Geometry: final body of the model. Coordinates: model frame, mm. A direction names the side the tool comes from. Round coordinates to 2 decimals unless told otherwise and drop trailing zeros. Loops run counter-clockwise (first coordinate to the right, second up) from the corner with the lowest first, then second, coordinate; pieces in that order, holes last. Notation, with made-up numbers: M -21,21 L -12,21 A33 ccw -12,53 Z; hole C 26,2 d8. An arc over 180 degrees is marked long. Answer as a JSON object with one key per item and string values.
from build123d import *

# Parameters (mm, degrees)
SKETCH1_W               = 35
SKETCH1_H               = 12.2
BOSS_EXTRUDE1_DEPTH     = 4
SKETCH2_R               = 1
CUT_EXTRUDE1_DEPTH      = 38.656658625
SKETCH3_W               = 10
SKETCH3_H               = 12.2
BOSS_EXTRUDE2_DEPTH     = 15
SKETCH4_W               = 12.2
SKETCH4_H               = 4
BOSS_EXTRUDE3_DEPTH     = 24
CUT_EXTRUDE2_DEPTH      = 42.133377247
CUT_EXTRUDE2_DEPTH_BACK = 42.133377247
SKETCH5_R               = 1
CUT_EXTRUDE3_DEPTH      = 0.5
CHAMFER1_SIZE           = 1.2
CUT_EXTRUDE17_DEPTH     = 2
CUT_EXTRUDE18_DEPTH     = 2
SKETCH26_W              = 5
SKETCH26_H              = 14
CUT_EXTRUDE19_DEPTH     = 43.113593099
CHAMFER2_SIZE           = 0.5


with BuildPart() as part:
    # Sketch1 → Boss-Extrude1 (new body)
    with BuildSketch(Plane.XY):
        with Locations((-18.048765432, 5.660493827)):
            Rectangle(SKETCH1_W, SKETCH1_H)
    extrude(amount=BOSS_EXTRUDE1_DEPTH)

    # Sketch2 → Cut-Extrude1 (cut, through all)
    with BuildSketch(Plane.XY.offset(4)):
        with Locations((-29.048765432, 5.660493827)):
            Circle(SKETCH2_R)
    extrude(amount=-CUT_EXTRUDE1_DEPTH, mode=Mode.SUBTRACT)

    # Sketch3 → Boss-Extrude2 (add)
    with BuildSketch(Plane.XY.offset(4)):
        with Locations((-5.548765432, 5.660493827)):
            Rectangle(SKETCH3_W, SKETCH3_H)
    extrude(amount=BOSS_EXTRUDE2_DEPTH)

    # Sketch4 → Boss-Extrude3 (add)
    with BuildSketch(Plane(origin=(-0.548765432, 0, 0), x_dir=(0, 0, -1), z_dir=(1, 0, 0))):
        with Locations((-12.9, 9.760493827)):
            Rectangle(SKETCH4_W, SKETCH4_H)
    extrude(amount=BOSS_EXTRUDE3_DEPTH)

    # Sketch5 → Cut-Extrude2 (cut, two sides: drawn at the far end of the back side and taken through both)
    with BuildSketch(Plane.XZ.offset(-7.760493827).offset(-CUT_EXTRUDE2_DEPTH_BACK)):
        with Locations(Location((16.951234568, 12.9, 0), (0, 0, 270))):
            Circle(SKETCH5_R)
        with Locations(Location((8.451234568, 12.9, 0), (0, 0, 270))):
            Circle(SKETCH5_R)
    extrude(amount=CUT_EXTRUDE2_DEPTH + CUT_EXTRUDE2_DEPTH_BACK, mode=Mode.SUBTRACT)

    # Sketch7 → Cut-Extrude3 (cut)
    with BuildSketch(Plane(origin=(0, 0, 0), x_dir=(-1, 0, 0), z_dir=(0, 0, -1))):
        Polygon((23.048765432, 5.660493827), (19.298765432, 7.825557337), (19.298765432, 3.495430318), align=None)
    extrude(amount=-CUT_EXTRUDE3_DEPTH, mode=Mode.SUBTRACT)

    # Chamfer1
    chamfer1_edges = [part.edges().sort_by_distance(p)[0] for p in [
        (-10.548765432, -0.439506173, 11.5),
        (-10.548765432, 5.660493827, 19),
        (-5.548765432, -0.439506173, 19),
        (23.451234568, 7.760493827, 12.9),
        (-0.548765432, 5.660493827, 0),
        (-18.048765432, -0.439506173, 0),
        (-35.548765432, 5.660493827, 0),
        (-0.548765432, -0.439506173, 9.5),
    ]]
    chamfer(chamfer1_edges, length=CHAMFER1_SIZE)

    # Sketch24 → Cut-Extrude17 (cut)
    with BuildSketch(Plane.XY.offset(4)):
        with BuildLine():
            Line((-27.048765432, 2.727491952), (-14.648765432, 3.660493827))
            ThreePointArc((-14.648765432, 3.660493827), (-12.648765432, 5.660493827), (-14.648765432, 7.660493827))
            Line((-14.648765432, 7.660493827), (-27.048765432, 8.593495702))
            ThreePointArc((-27.048765432, 8.593495702), (-32.598765432, 5.660493827), (-27.048765432, 2.727491952))
        make_face()
    extrude(amount=-CUT_EXTRUDE17_DEPTH, mode=Mode.SUBTRACT)

    # Sketch25 → Cut-Extrude18 (cut)
    with BuildSketch(Plane.XZ.offset(-7.760493827)):
        with BuildLine():
            Line((2.551234568, 14.9), (14.951234568, 15.833001875))
            ThreePointArc((14.951234568, 15.833001875), (20.501234568, 12.9), (14.951234568, 9.966998125))
            Line((14.951234568, 9.966998125), (2.551234568, 10.9))
            ThreePointArc((2.551234568, 10.9), (0.551234568, 12.9), (2.551234568, 14.9))
        make_face()
    extrude(amount=-CUT_EXTRUDE18_DEPTH, mode=Mode.SUBTRACT)

    # Sketch26 → Cut-Extrude19 (cut, through all)
    with BuildSketch(Plane(origin=(0, 11.760493827, 0), x_dir=(1, 0, 0), z_dir=(0, 1, 0))):
        with Locations((-5.548765432, -9.5)):
            Rectangle(SKETCH26_W, SKETCH26_H)
    extrude(amount=-CUT_EXTRUDE19_DEPTH, mode=Mode.SUBTRACT)

    # Chamfer2
    chamfer2_edges = [part.edges().sort_by_distance(p)[0] for p in [
        (-8.048765432, -0.439506173, 9.5),
        (-5.548765432, -0.439506173, 2.5),
        (-3.048765432, -0.439506173, 9.5),
        (-5.548765432, -0.439506173, 16.5),
        (-8.048765432, 11.760493827, 9.5),
        (-5.548765432, 11.760493827, 16.5),
        (-3.048765432, 11.760493827, 9.5),
        (-5.548765432, 11.760493827, 2.5),
    ]]
    chamfer(chamfer2_edges, length=CHAMFER2_SIZE)


solid = part.part
1) Section query B-B (y = 1.5). Return the cut outline in (x, z).
Results:
{"outline": "M -35.55,1.2 L -34.35,0 L -1.75,0 L -0.55,1.2 L -0.55,19 L -9.35,19 L -10.55,17.8 L -10.55,4 L -35.55,4 Z; hole M -8.05,2.5 L -3.05,2.5 L -3.05,16.5 L -8.05,16.5 Z"}
2) Reachability of faces 4 (the flat face through (-10.549, 6, 11)), 5 (the cylindrical face through (-12.65, 5.62, 3.01)), 6 (the flat face through (11, 10, 6.8)), 7 (the flat face through (11, 7.76, 16)) from +Z, -Z, +X, -X, +Y, -Y: full face, straight path, thin tool, end or side. Return the list, or none.
Results:
{"face 4": "+Z, -X, +Y, -Y", "face 5": "+Z", "face 6": "-Z, +X, +Y, -Y", "face 7": "+Z, -Z, +X, -Y"}
3) Ray query, line 1 (X direction, y = 5.25, z = 11); line 2 (X direction, y = 11.35, z = 12.9); line 3 (Y direction, x = 17.5, z = 14.25). Return the intervals inside material, ascending.
Results:
{"line 1": "-10.55 to -8.05, -3.05 to -0.55", "line 2": "-10.55 to -8.14, -2.96 to 7.45, 9.45 to 15.95, 17.95 to 23.45", "line 3": "9.76 to 11.76"}
4) Pin query (flat end, axial travel): P1, Ø1.5, axis at x = 11.5, y = 10, coming from the -Z side; P2, Ø5, axis at y = 4.5, z = 13, coming from the -X side; P3, Ø8, axis at x = 13, z = 13, coming from the -Y side. Return the tip coordinate at first contact, or that it passes through.
Results:
{"P1": "z = 6.8", "P2": "x = -10.55", "P3": "y = 7.76"}
5) Section query C-C (z = 5). Return the cut outline in (x, y), and give its area (3 significant figures).
Results:
{"outline": "M -10.55,0.76 L -9.35,-0.44 L -8.55,-0.44 L -8.05,0.06 L -8.05,11.26 L -8.55,11.76 L -10.55,11.76 Z; M -3.05,0.06 L -2.55,-0.44 L -1.75,-0.44 L -0.55,0.76 L -0.55,11.76 L -2.55,11.76 L -3.05,11.26 Z", "area": "59.1 mm2"}
6) Pull-direction query (X, two-part tool) for faces 1 (the flat face through (-18.89, 0.17, 0.59)), 2 (the flat face through (-1.14, 0.17, 9.98)), 3 (the flat face through (11, 9.76, 13)); classes: +X half, -X half, draft (parallel to the pull), parting line (faces both ways), or undercut.
Results:
{"face 1": "draft", "face 2": "+X half", "face 3": "undercut"}
7) Section query A-A (z = 12.9). Count the separate pieces of the cut face and the enclosed holes in it, and give its area (3 significant figures).
Results:
{"separate pieces": "4", "enclosed holes": "0", "area": "106 mm2"}
